Input: part model. Units: mm. Frame: model coordinates. A direction names the side the tool comes from. Round coordinates to 2 decimals unless told otherwise and drop trailing zeros. Write each loop counter-clockwise with the first axis right and the second up, starting at its lowest first coordinate (ties: lowest second). Pieces come first, ordered by that corner, then holes. Notation, with made-up numbers: (83.5, -20) - (88.5, -20) arc R20 cw to (88.5, -15) - close; hole circle Ø4 at (-35, 88). An arc over 180 degrees is marked (long way). One line per item, written item: value. Start each with the question number.
```python
from build123d import *

# Parameters (mm, degrees)
SKETCH1_W           = 70
SKETCH1_H           = 30
BOSS_EXTRUDE1_DEPTH = 3
SKETCH2_R           = 1.5
SKETCH2_R_2         = 2
CUT_EXTRUDE2_DEPTH  = 4


with BuildPart() as part:
    # Sketch1 → Boss-Extrude1 (new body)
    with BuildSketch(Plane.XY):
        Rectangle(SKETCH1_W, SKETCH1_H)
    extrude(amount=BOSS_EXTRUDE1_DEPTH)

    # Sketch2 → Cut-Extrude2 (cut, through all)
    with BuildSketch(Plane.XY.offset(3)):
        with Locations((32, 12)):
            Circle(SKETCH2_R)
        with Locations((-32, 12)):
            Circle(SKETCH2_R)
        with Locations((32, -12)):
            Circle(SKETCH2_R)
        with Locations((-32, -12)):
            Circle(SKETCH2_R)
        with Locations((-11, 0)):
            Circle(SKETCH2_R_2)
        with Locations((-31, 0)):
            Circle(SKETCH2_R_2)
        with Locations((14, 0)):
            Circle(SKETCH2_R_2)
        with BuildLine():
            Line((-29.032472505, 12.440205142), (-12.8, 12.440205142))
            Line((-12.8, 12.440205142), (-12.8, 3.57211422))
            ThreePointArc((-12.8, 3.57211422), (-14.054873196, 2.582198629), (-14.821990136, 1.179996355))
            Line((-14.821990136, 1.179996355), (-27.178009864, 1.179996355))
            ThreePointArc((-27.178009864, 1.179996355), (-27.884686293, 2.508948087), (-29.032472505, 3.48264778))
            Line((-29.032472505, 3.48264778), (-29.032472505, 11.559794858))
            ThreePointArc((-29.032472505, 11.559794858), (-29, 12), (-29.032472505, 12.440205142))
        make_face()
        with BuildLine():
            Line((11.174466994, 2.831318285), (-8.174466994, 2.831318285))
            ThreePointArc((-8.174466994, 2.831318285), (-8.703062454, 3.274763794), (-9.3, 3.620773398))
            Line((-9.3, 3.620773398), (-9.3, 12))
            Line((-9.3, 12), (12.3, 12))
            Line((12.3, 12), (12.3, 3.620773398))
            ThreePointArc((12.3, 3.620773398), (11.703062454, 3.274763794), (11.174466994, 2.831318285))
        make_face()
        with BuildLine():
            Line((30, 1.179996355), (17.821990136, 1.179996355))
            ThreePointArc((17.821990136, 1.179996355), (17.054873196, 2.582198629), (15.8, 3.57211422))
            Line((15.8, 3.57211422), (15.8, 12))
            Line((15.8, 12), (29, 12))
            ThreePointArc((29, 12), (29.261387212, 10.775255129), (30, 9.763932023))
            Line((30, 9.763932023), (30, 1.179996355))
        make_face()
    cut_extrude2 = extrude(amount=-CUT_EXTRUDE2_DEPTH, mode=Mode.SUBTRACT)

    # Mirror1: Cut-Extrude2 across plane
    add(cut_extrude2.mirror(Plane.ZX), mode=Mode.SUBTRACT)


solid = part.part
```
Q1. Material intervals for probe 1 along Y at (x, z) = (-24.5, 0.5); probe 2 along X at (y, z) = (-9.5, 2.4); probe 3 along Y at (x, z) = (1, 2.25), sorted ascending. Write a range as from..to.
Q2. Cut plane B-B, the plane y = 0. Output: boundary loops of the cut face in (x, z), and give its area (3 significant figures).
Q3. Contact query for a flat-ended pin moving along its axis: pin 1 Ø2.5 at (x, y) = (32, -12) entering from -Z. Output: stop coordinate, or through.
Q4. Cut plane C-C, the plane x = -11. Output: boundary loops of the cut face in (y, z), and give its area (3 significant figures).
Q5. Pull-direction query (X, two-part tool) for faces 1 (the flat face through (-29.032, -7, 2)), 2 (the flat face through (0, 0, 3)); classes: pulls with the +X half, pulls with the -X half, needs draft (parallel to the pull), parting line crosses it, or undercut.
Q6. Access query for faces 3 (the flat face through (0, 0, 0)), 4 (the cylindrical face through (29.254, 10.791, 1.521)). Directions: +Z, -Z, +X, -X, +Y, -Y. A direction counts if a zero-diameter tool reaches every point of the face in a straight line with its end or side. Return the directions, or none.
Q7. Cut plane D-D, the plane y = -7.25. Output: boundary loops of the cut face in (x, z).
Q8. Cut plane A-A, the plane x = 22.5. Output: boundary loops of the cut face in (y, z), and give its area (3 significant figures).
A:
1. probe 1: y = -15..-12.44, -1.18..1.18, 12.44..15
1. probe 2: x = -35..-29.03, -12.8..-9.3, 12.3..15.8, 30..35
1. probe 3: y = -15..-12, -2.83..2.83, 12..15
2. outline: (-35, 0) - (-33, 0) - (-33, 3) - (-35, 3) - close; (-29, 0) - (-13, 0) - (-13, 3) - (-29, 3) - close; (-9, 0) - (12, 0) - (12, 3) - (-9, 3) - close; (16, 0) - (35, 0) - (35, 3) - (16, 3) - close
2. area: 174 mm²
3. pin 1: passes through
4. outline: (-15, 0) - (-2, 0) - (-2, 3) - (-15, 3) - close; (2, 0) - (15, 0) - (15, 3) - (2, 3) - close
4. area: 78.0 mm²
5. face 1: undercut
5. face 2: needs draft
6. face 3: -Z, +X, -X, +Y, -Y
6. face 4: +Z, -Z
7. outline: (-35, 0) - (-29.03, 0) - (-29.03, 3) - (-35, 3) - close; (-12.8, 0) - (-9.3, 0) - (-9.3, 3) - (-12.8, 3) - close; (12.3, 0) - (15.8, 0) - (15.8, 3) - (12.3, 3) - close; (30, 0) - (35, 0) - (35, 3) - (30, 3) - close
8. outline: (-15, 0) - (-12, 0) - (-12, 3) - (-15, 3) - close; (-1.18, 0) - (1.18, 0) - (1.18, 3) - (-1.18, 3) - close; (12, 0) - (15, 0) - (15, 3) - (12, 3) - close
8. area: 25.1 mm²
